```python
from build123d import *

# Parameters (mm, degrees)
BOSS_EXTRUDE1_DEPTH      = 10
BOSS_EXTRUDE1_DEPTH_BACK = 10
SKETCH2_W                = 14
SKETCH2_H                = 20
BOSS_EXTRUDE2_DEPTH      = 10
CUT_EXTRUDE1_DEPTH       = 5.2
CUT_EXTRUDE2_DEPTH       = 20


with BuildPart() as part:
    # Sketch1 → Boss-Extrude1 (new, two sides: drawn at the far end of the back side and taken through both)
    with BuildSketch(Plane.XY.offset(-BOSS_EXTRUDE1_DEPTH_BACK)):
        Polygon((-55, 21.875), (55, -5.625), (55, -8.125), (-55, -8.125), align=None)
    extrude(amount=BOSS_EXTRUDE1_DEPTH + BOSS_EXTRUDE1_DEPTH_BACK)

    # Sketch2 → Boss-Extrude2 (add)
    with BuildSketch(Plane(origin=(1.911764706, 7.647058824, 0), x_dir=(0.970142500145332, -0.24253562503633289, 0), z_dir=(0.24253562503633289, 0.970142500145332, 0))):
        Polygon((-53.463304306, -10), (-38.463304306, -10), (-38.463304306, -0.564895404), (-45.408034785, -5.450442479), (-53.463304306, 6), align=None)
        with Locations((13.286695694, 0)):
            Rectangle(SKETCH2_W, SKETCH2_H)
    extrude(amount=BOSS_EXTRUDE2_DEPTH)

    # Sketch3 → Cut-Extrude1 (cut)
    with BuildSketch(Plane.XZ.offset(8.125)):
        Polygon((15.692093342, 10.058542854), (14.11294757, 4.9), (22.553719096, 4.9), (20.974573324, 10.058542854), align=None)
        Polygon((-20.974573324, 10.058542854), (-22.553719096, 4.9), (-14.11294757, 4.9), (-15.692093342, 10.058542854), align=None)
    extrude(amount=-CUT_EXTRUDE1_DEPTH, mode=Mode.SUBTRACT)

    # Sketch4 → Cut-Extrude2 (cut)
    with BuildSketch(Plane.XY.offset(10)):
        Polygon((9.829772572, 13.398379905), (10.436111635, 15.823736155), (24.018106637, 12.428237405), align=None)
    extrude(amount=-CUT_EXTRUDE2_DEPTH, mode=Mode.SUBTRACT)


solid = part.part
```
Work out the finished part from the listing and answer in its coordinate system (mm). A direction names the side the tool comes from. Round coordinates to 2 decimals unless told otherwise and drop trailing zeros. Loops run counter-clockwise (first coordinate to the right, second up) from the corner with the lowest first, then second, coordinate; pieces in that order, holes last.
(1) Each of these flat-tipped pins is pushed along its axis until it touches: P1, Ø1.5, axis at x = -17, z = 8.5, coming from the -Y side (3 decimals); P2, Ø5, axis at x = 14.5, z = -3, coming from the +Y side. Where does it stop, or does it pass through?
Computed values:
P1: stops at y = -2.925
P2: stops at y = 13.25
(2) The part is cut by section C-C, the plane x = -23.5. Give the vertices of the cut face in (y, z) (3 decimals).
Computed values:
outline: (-8.125, -10) - (14, -10) - (14, 10) - (-8.125, 10) - close
(3) The part is cut by section D-D, the plane y = 16. Give the vertices of the cut face in (x, z).
Computed values:
outline: (-55, -10) - (-31.5, -10) - (-31.5, 10) - (-55, 10) - close
(4) The mould has two halves that part along Z. Classify faces 1 (the flat face through (-18, -2.925, 7)), 2 (the flat face through (-23.9, 14.1, -0.1)), 3 (the flat face through (-11, 3, 10)): pulls with the +Z half, pulls with the -Z half, needs draft (parallel to the pull), parting line crosses it, or undercut.
Computed values:
face 1: undercut
face 2: needs draft
face 3: pulls with the +Z half
(5) For faces 4 (the flat face through (8.908, 9.709, 0.14)), 5 (the flat face through (18, -6, 4.9)), 6 (the flat face through (-37.529, 22.589, 2.973)), determine the directions among +Z, -Z, +X, -X, +Y, -Y from which every point of the face is accessible in a straight line to the end or side of a thin tool.
Computed values:
face 4: +Z, -Z, +Y
face 5: -Y
face 6: -Z
(6) The part is cut by section B-B, the plane z = -5. Give the vertices of the cut face in (x, y) (3 decimals), and give its area (3 significant figures).
Computed values:
outline: (-55, -8.125) - (55, -8.125) - (55, -5.625) - (21.593, 2.727) - (24.018, 12.428) - (9.83, 13.398) - (8.011, 6.122) - (-49.273, 20.443) - (-46.847, 30.145) - (-47.53, 30.315) - (-49.955, 20.614) - (-55, 21.875) - close
area: 1,920 mm2
(7) Find the intervals of material crossed by L1, parallel to X at y = 25.5, z = 3; L2, parallel to Y at x = 43.5, z = 4 (3 decimals); L3, parallel to X at y = 25, z = 5.5, in increasing order.
Computed values:
L1: x = -48.73 to -42.21, -36.84 to -33.27
L2: y = -8.125 to -2.75
L3: x = -48.86 to -33.4
(8) The part is cut by section A-A, the plane y = 10. Give the vertices of the cut face in (x, z), and give its area (3 significant figures).
Computed values:
outline: (-55, -10) - (-7.5, -10) - (-7.5, 10) - (-55, 10) - close; (8.98, -10) - (23.41, -10) - (23.41, 10) - (8.98, 10) - close
area: 1,240 mm2
